Source: CAD feature listing. Evaluate the final solid. Frame: model axes, mm. Give positions to 0.01 mm unless a question says otherwise; leave off trailing zeros. Loops run counter-clockwise (first coordinate to the right, second up) from the corner with the lowest first, then second, coordinate; pieces in that order, holes last.
```python
from build123d import *

# Parameters (mm, degrees)
BOSS_EXTRUDE1_DEPTH = 4
CUT_EXTRUDE1_REACH  = 33.978
SKETCH2_R           = 1.6


with BuildPart() as part:
    # Sketch1 → Boss-Extrude1 (new body)
    with BuildSketch(Plane.XY):
        with BuildLine():
            Line((-14, 20.75), (14, 20.75))
            ThreePointArc((14, 20.75), (21.071067812, 17.821067812), (24, 10.75))
            Line((24, 10.75), (24, -10.75))
            ThreePointArc((24, -10.75), (21.071067812, -17.821067812), (14, -20.75))
            Line((14, -20.75), (-14, -20.75))
            ThreePointArc((-14, -20.75), (-21.071067812, -17.821067812), (-24, -10.75))
            Line((-24, -10.75), (-24, 10.75))
            ThreePointArc((-24, 10.75), (-21.071067812, 17.821067812), (-14, 20.75))
        make_face()
    extrude(amount=BOSS_EXTRUDE1_DEPTH)

    # Sketch2 → Cut-Extrude1 (cut, up to next)
    with BuildSketch(Plane.XY, mode=Mode.PRIVATE) as cut_extrude1_sk1:
        with Locations((-7, -17.25)):
            Circle(SKETCH2_R)
    cut_extrude1_tool1 = extrude(cut_extrude1_sk1.sketch, amount=CUT_EXTRUDE1_REACH, mode=Mode.PRIVATE) & part.part
    # Sketch2 → Cut-Extrude1 (cut, up to next)
    with BuildSketch(Plane.XY, mode=Mode.PRIVATE) as cut_extrude1_sk2:
        with Locations((-7, 17.25)):
            Circle(SKETCH2_R)
    cut_extrude1_tool2 = extrude(cut_extrude1_sk2.sketch, amount=CUT_EXTRUDE1_REACH, mode=Mode.PRIVATE) & part.part
    # Sketch2 → Cut-Extrude1 (cut, up to next)
    with BuildSketch(Plane.XY, mode=Mode.PRIVATE) as cut_extrude1_sk3:
        with Locations((18.5, -5.8)):
            Circle(SKETCH2_R)
    cut_extrude1_tool3 = extrude(cut_extrude1_sk3.sketch, amount=CUT_EXTRUDE1_REACH, mode=Mode.PRIVATE) & part.part
    # Sketch2 → Cut-Extrude1 (cut, up to next)
    with BuildSketch(Plane.XY, mode=Mode.PRIVATE) as cut_extrude1_sk4:
        with Locations((18.5, 1.3)):
            Circle(SKETCH2_R)
    cut_extrude1_tool4 = extrude(cut_extrude1_sk4.sketch, amount=CUT_EXTRUDE1_REACH, mode=Mode.PRIVATE) & part.part
    # Sketch2 → Cut-Extrude1 (cut, up to next)
    with BuildSketch(Plane.XY, mode=Mode.PRIVATE) as cut_extrude1_sk5:
        with Locations((-18.5, -5.8)):
            Circle(SKETCH2_R)
    cut_extrude1_tool5 = extrude(cut_extrude1_sk5.sketch, amount=CUT_EXTRUDE1_REACH, mode=Mode.PRIVATE) & part.part
    # Sketch2 → Cut-Extrude1 (cut, up to next)
    with BuildSketch(Plane.XY, mode=Mode.PRIVATE) as cut_extrude1_sk6:
        with Locations((-18.5, 1.3)):
            Circle(SKETCH2_R)
    cut_extrude1_tool6 = extrude(cut_extrude1_sk6.sketch, amount=CUT_EXTRUDE1_REACH, mode=Mode.PRIVATE) & part.part
    add(cut_extrude1_tool1.solids().sort_by_distance((-7, -17.25, 0))[0], mode=Mode.SUBTRACT)
    add(cut_extrude1_tool2.solids().sort_by_distance((-7, 17.25, 0))[0], mode=Mode.SUBTRACT)
    add(cut_extrude1_tool3.solids().sort_by_distance((18.5, -5.8, 0))[0], mode=Mode.SUBTRACT)
    add(cut_extrude1_tool4.solids().sort_by_distance((18.5, 1.3, 0))[0], mode=Mode.SUBTRACT)
    add(cut_extrude1_tool5.solids().sort_by_distance((-18.5, -5.8, 0))[0], mode=Mode.SUBTRACT)
    add(cut_extrude1_tool6.solids().sort_by_distance((-18.5, 1.3, 0))[0], mode=Mode.SUBTRACT)


solid = part.part
```
(1) Ray query, line 1 along Y through (x, z) = (-7, 2.5); line 2 along X through (y, z) = (-5.8, 2.85); line 3 along Y through (x, z) = (18.5, 2.75). Return the intervals inside material, ascending.
A:
line 1: y = -20.75 to -18.85, -15.65 to 15.65, 18.85 to 20.75
line 2: x = -24 to -20.1, -16.9 to 16.9, 20.1 to 24
line 3: y = -19.68 to -7.4, -4.2 to -0.3, 2.9 to 19.68
(2) Section B-B, the plane z = 2.9. Return the cut outline in (x, y), then the cut area to 3 significant figures.
A:
outline: (-24, -10.75) arc R10 ccw to (-14, -20.75) - (14, -20.75) arc R10 ccw to (24, -10.75) - (24, 10.75) arc R10 ccw to (14, 20.75) - (-14, 20.75) arc R10 ccw to (-24, 10.75) - close; hole circle Ø3.2 at (-18.5, -5.8); hole circle Ø3.2 at (-18.5, 1.3); hole circle Ø3.2 at (-7, -17.25); hole circle Ø3.2 at (-7, 17.25); hole circle Ø3.2 at (18.5, -5.8); hole circle Ø3.2 at (18.5, 1.3)
area: 1,860 mm2
(3) Section D-D, the plane y = -17.25. Return the cut outline in (x, z), then the cut area to 3 significant figures.
A:
outline: (-21.6, 0) - (-8.6, 0) - (-8.6, 4) - (-21.6, 4) - close; (-5.4, 0) - (21.6, 0) - (21.6, 4) - (-5.4, 4) - close
area: 160 mm2
(4) Section C-C, the plane x = -7. Return the cut outline in (y, z).
A:
outline: (-20.75, 0) - (-18.85, 0) - (-18.85, 4) - (-20.75, 4) - close; (-15.65, 0) - (15.65, 0) - (15.65, 4) - (-15.65, 4) - close; (18.85, 0) - (20.75, 0) - (20.75, 4) - (18.85, 4) - close
(5) Mould query, pull axis Y, two halves, no side actions, for faces 1 (the cylindrical face through (-19.68, -4.72, 1.97)), 2 (the flat face through (0, 20.75, 2)), 3 (the cylindrical face through (17.32, -4.72, 1.97)), 4 (the flat face through (24, 0, 2)). Classes: pulls with the +Y half, pulls with the -Y half, needs draft (parallel to the pull), parting line crosses it, or undercut.
A:
face 1: undercut
face 2: pulls with the +Y half
face 3: undercut
face 4: needs draft
(6) Section A-A, the plane y = 1.3. Return the cut outline in (x, z), then the cut area to 3 significant figures.
A:
outline: (-24, 0) - (-20.1, 0) - (-20.1, 4) - (-24, 4) - close; (-16.9, 0) - (16.9, 0) - (16.9, 4) - (-16.9, 4) - close; (20.1, 0) - (24, 0) - (24, 4) - (20.1, 4) - close
area: 166 mm2
